Source: CAD feature listing. Evaluate the final solid. Frame: model axes, mm. Give positions to 0.01 mm unless a question says otherwise; leave off trailing zeros. Order: outer loops, then holes, each group sorted by start corner. A loop starts at its lowest first (then second) coordinate and runs counter-clockwise, first axis right, second up. Notation, with made-up numbers: (31.5, 31.5) -> (55.5, 31.5) arc R28 ccw to (55.5, 53.5) -> close; hole circle Ø2 at (84.5, 64). An arc over 180 degrees is marked (long way). Answer in a Markdown table with one row per item.
Autodesk Inventor part; units mm, degrees
ref_plane "YZ Plane" through (0, 0, 0) normal (1, 0, 0) x (0, 1, 0)
ref_plane "XZ Plane" through (0, 0, 0) normal (0, 1, 0) x (-1, 0, 0)
ref_plane "XY Plane" through (0, 0, 0) normal (0, 0, 1) x (1, 0, 0)
sketch "Boceto principal" plane through (0, 0, 0) normal (1, 0, 0) x (0, 1, 0)
  line L0 (0, -1) -> (0, -3)
  line L1 (0, -3) -> (2, -3)
  line L2 (2, -3) -> (2, -2)
  line L3 (2, -2) -> (6, -2)
  line L4 (7, -3) -> (7, -27)
  line L5 (6, -28) -> (2, -28)
  line L6 (2, -28) -> (2, -27)
  line L7 (2, -27) -> (0, -27)
  line L8 (0, -27) -> (0, -29)
  line L9 (1, -30) -> (8, -30)
  line L10 (9, -29) -> (9, -1)
  line L11 (8, 0) -> (1, 0)
  arc A0 (1, 0) -> (0, -1) centre (1, -1) ccw
  arc A1 (7, -3) -> (6, -2) centre (6, -3) ccw
  arc A2 (6, -28) -> (7, -27) centre (6, -27) ccw
  arc A3 (0, -29) -> (1, -30) centre (1, -29) ccw
  arc A4 (8, -30) -> (9, -29) centre (8, -29) ccw
  arc A5 (9, -1) -> (8, 0) centre (8, -1) ccw
extrude "Extrusion1" add sketch "Boceto principal" along normal blind 438
sketch "Boceto esquinas" plane through (0, 0, 0) normal (0, 1, 0) x (-1, 0, 0)
  line L0 (0, 0) -> (-30, 0)
  line L1 (-30, 0) -> (0, -30)
  line L2 (0, -30) -> (0, 0)
  line L3 (-408, 0) -> (-438, 0)
  line L4 (-438, 0) -> (-438, -30)
  line L5 (-438, -30) -> (-408, 0)
extrude "Extrusion2" cut sketch "Boceto esquinas" along normal blind 10
properties part number "Tapa 30x30 438mm" material "PVC, Flexible"
(1) Section query C-C (z = -16.5). Return the cut outline in (x, y).
A:
| item | result |
|---|---|
| outline | (13.5, 7) -> (424.5, 7) -> (424.5, 9) -> (13.5, 9) -> close |
(2) First-contact query: pin 1 Ø4.5 at (x, y) = (196.5, 4.5) entering from +Z; pin 2 Ø1.5 at (x, z) = (148.5, -10) entering from -Y. Flat tips, straight axial feed; report the tip coordinate or a pass-through.
A:
| item | result |
|---|---|
| pin 1 | stops at z = 0 |
| pin 2 | stops at y = 7 |
(3) Pull-direction query (Z, two-part tool) for faces 1 (the flat face through (216, 4, -30)), 2 (the flat face through (216, 7, -15)), 3 (the flat face through (423.2, 7.4, -15.2)); classes: +Z half, -Z half, draft (parallel to the pull), parting line (faces both ways), or undercut.
A:
| item | result |
|---|---|
| face 1 | -Z half |
| face 2 | undercut |
| face 3 | +Z half |
(4) Section query B-B (x = 75). Return the cut outline in (y, z), plus the area to 3 significant figures.
A:
| item | result |
|---|---|
| outline | (0, -29) arc R1 ccw to (1, -30) -> (8, -30) arc R1 ccw to (9, -29) -> (9, -1) arc R1 ccw to (8, 0) -> (1, 0) arc R1 ccw to (0, -1) -> (0, -3) -> (2, -3) -> (2, -2) -> (6, -2) arc R1 cw to (7, -3) -> (7, -27) arc R1 cw to (6, -28) -> (2, -28) -> (2, -27) -> (0, -27) -> close |
| area | 91.6 mm^2 |
(5) Ray query, probe 1 along Z at (x, y) = (327, 2.25); probe 2 along Z at (x, y) = (386, 1.5); probe 3 along Y at (x, z) = (267, -21). Return the intervals inside material, ascending.
A:
| item | result |
|---|---|
| probe 1 | z = -30 to -28, -2 to 0 |
| probe 2 | z = -30 to -27, -3 to 0 |
| probe 3 | y = 7 to 9 |
(6) Section query A-A (y = 3.5). Return the cut outline in (x, z).
A:
| item | result |
|---|---|
| outline | (0, -30) -> (438, -30) -> (436, -28) -> (2, -28) -> close; (28, -2) -> (410, -2) -> (408, 0) -> (30, 0) -> close |
